Geometry: see drawing. Coordinates: mm, zero at the bounding-box minimum. A direction names the side the tool comes from. Coordinates: 2 decimals unless noted, no trailing zeros. Write each loop counter-clockwise with the first axis right and the second up, starting at its lowest first coordinate (ties: lowest second). Pieces come first, ordered by that corner, then holes. Notation, with made-up numbers: (39.5, 23) - (77.5, 23) arc R23 ccw to (77.5, 42) - close; hole circle Ø9 at (6, 2.25). An arc over 180 degrees is marked (long way). One line per question, with ' | ' between items. Start each with the question number.
1) Section query B-B on z = 50. Return loops of the section in (x, y), and give its area (3 significant figures).
2) Reachability of the marked faces 1, 2 and 3 from +Z, -Z, +X, -X, +Y, -Y: full face, straight path, thin tool, end or side. Return the list, or none.
3) Section query D-D on y = 21.5. Return loops of the section in (x, z), and give its area (3 significant figures).
4) Section query C-C on x = 13. Return loops of the section in (y, z).
5) Draft query along X for the marked faces 4, 5 and 6. Return one class per face: released by +X, released by -X, zero draft, split by the parting line, or undercut.
6) Line query: line 1 (Z direction, x = 65, y = 45); line 2 (X direction, y = 17, z = 10); line 3 (Y direction, x = 108, z = 95). Output: solid intervals per line, ascending.
7) Section query A-A on y = 45. Return loops of the section in (x, z).
8) First-contact query: P1, Ø2, axis at x = 97, z = 12, coming from the -Y side; P2, Ø2, axis at x = 59, z = 36, coming from the +Y side; P3, Ø12, axis at x = 82, y = 79, coming from the -Z side. Flat tips, straight axial feed; report the tip coordinate or a pass-through.
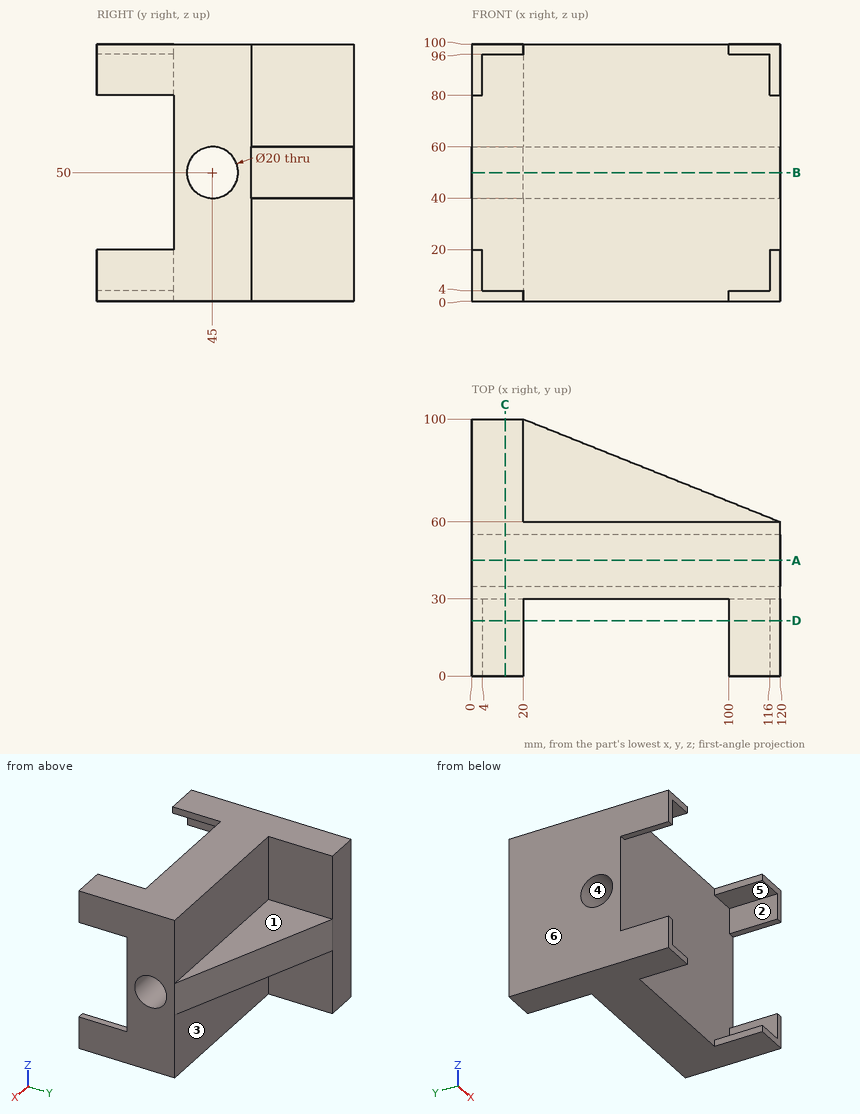
Answer key:
1) outline: (0, 30) - (120, 30) - (120, 35) - (0, 35) - close; (0, 55) - (120, 55) - (120, 60) - (20, 100) - (0, 100) - close | area: 4,000 mm²
2) face 1: +Z, +X, +Y | face 2: -Y | face 3: -Z, +X, +Y
3) outline: (0, 0) - (20, 0) - (20, 4) - (4, 4) - (4, 20) - (0, 20) - close; (0, 80) - (4, 80) - (4, 96) - (20, 96) - (20, 100) - (0, 100) - close; (100, 0) - (120, 0) - (120, 20) - (116, 20) - (116, 4) - (100, 4) - close; (100, 96) - (116, 96) - (116, 80) - (120, 80) - (120, 100) - (100, 100) - close | area: 576 mm²
4) outline: (0, 0) - (100, 0) - (100, 100) - (0, 100) - (0, 96) - (30, 96) - (30, 4) - (0, 4) - close; hole circle Ø20 at (45, 50)
5) face 4: zero draft | face 5: undercut | face 6: released by -X
6) line 1: 0 to 40, 60 to 100 | line 2: 0 to 4, 116 to 120 | line 3: 30 to 60
7) outline: (0, 0) - (120, 0) - (120, 40) - (0, 40) - close; (0, 60) - (120, 60) - (120, 100) - (0, 100) - close
8) P1: y = 30 | P2: y = 60 | P3: z = 40
